For this review, take the finished solid that the model builds, in its own axes (mm). A direction names the side the tool comes from. Coordinates: 2 decimals unless noted, no trailing zeros. Loops run counter-clockwise (first coordinate to the right, second up) from the corner with the lowest first, then second, coordinate; pieces in that order, holes last. Notation, with made-up numbers: (61, -9.75) - (68, -9.75) arc R30 cw to (68, 19.25) - close; hole circle Ø4 at (-5.5, 17.25). An arc over 180 degrees is marked (long way). One line per item, written item: value. Start each with the question number.
1. To check wall thickness, follow line 1 (Y direction, x = 0.25, z = 0); line 2 (X direction, y = 3, z = -10); line 3 (X direction, y = 5, z = -1.5). State the ranges of each line that lie inside material, in increasing order. Write a range as from..to.
2. The part is to be moulded in two halves that separate along Z. For faces 4 (the face through (10.8, 17.25, 2.27)), 5 (the face through (0.49, 6.31, 20.03)), 6 (the face through (0, -20, 7)), say which applies: released by +Z, released by -Z, zero draft, split by the parting line, or undercut.
3. For faces 1 (the face through (2, 0, 0)), 2 (the face through (17, 0, 0)), 3 (the face through (13.479, 8.923, 1.172)), list the 3-axis set-ups (+Z, -Z, +X, -X, +Y, -Y) from which the entire face can be reached by the end or side of a thin tool; tool diameter is ignored.
4. Take a section at B-B, the plane x = 10.5. State the section outline as (y, z) points, and give its area (3 significant figures).
5. Take a section at A-A, the plane z = 0. State the section outline as (x, y) points.
6. Insertion check: pin 1 (6 mm diameter, centred on x = 2.5, y = -9.5, fed in from -Z); pin 2 (4 mm diameter, centred on x = 9, z = 5, fed in from -Y); pin 3 (2 mm diameter, centred on y = -17, z = 2.5, fed in from -X). Each pin has a flat end and moves straight along its axis. Give the tip position at first contact, or say it passes through.
```python
from build123d import *

# Parameters (mm, degrees)
SKETCH1_R           = 22.5
BOSS_EXTRUDE1_DEPTH = 3
SKETCH3_R           = 17
SKETCH2_R           = 20
SKETCH4_R           = 9
BOSS_EXTRUDE2_DEPTH = 5
FILLET1_R           = 2
FILLET2_R           = 1
SKETCH5_R           = 21
CUT_EXTRUDE1_DEPTH  = 2
BOSS_EXTRUDE3_START = 1
SKETCH6_R           = 21
SKETCH6_R_2         = 16
BOSS_EXTRUDE3_DEPTH = 1
FILLET3_R           = 6


with BuildPart() as part:
    # Sketch1 → Boss-Extrude1 (new body)
    with BuildSketch(Plane(origin=(0, 0, 0), x_dir=(0, 0, -1), z_dir=(1, 0, 0))):
        Circle(SKETCH1_R)
    extrude(amount=BOSS_EXTRUDE1_DEPTH)

    # Sketch3 → Loft1 section 0
    with BuildSketch(Plane(origin=(12, 0, 0), x_dir=(0, 0, -1), z_dir=(1, 0, 0))):
        Circle(SKETCH3_R)
    # Sketch2 → Loft1 section 1
    with BuildSketch(Plane(origin=(3, 0, 0), x_dir=(0, 0, -1), z_dir=(1, 0, 0))):
        Circle(SKETCH2_R)
    loft()

    # Sketch4 → Boss-Extrude2 (add)
    with BuildSketch(Plane(origin=(12, 0, 0), x_dir=(0, 0, -1), z_dir=(1, 0, 0))):
        Circle(SKETCH4_R)
    extrude(amount=BOSS_EXTRUDE2_DEPTH)

    # Fillet1
    fillet1_edges = [part.edges().sort_by_distance(p)[0] for p in [
        (17, 0, 9),
    ]]
    fillet(fillet1_edges, radius=FILLET1_R)

    # Fillet2
    fillet2_edges = [part.edges().sort_by_distance(p)[0] for p in [
        (3, 0, 22.5),
        (12, 0, 17),
    ]]
    fillet(fillet2_edges, radius=FILLET2_R)

    # Sketch5 → Cut-Extrude1 (cut)
    with BuildSketch(Plane.ZY):
        Circle(SKETCH5_R)
    extrude(amount=-CUT_EXTRUDE1_DEPTH, mode=Mode.SUBTRACT)

    # Sketch6 → Boss-Extrude3 (add)
    with BuildSketch(Plane.ZY.offset(-2).offset(BOSS_EXTRUDE3_START)):
        Circle(SKETCH6_R)
        Circle(SKETCH6_R_2, mode=Mode.SUBTRACT)
    extrude(amount=-BOSS_EXTRUDE3_DEPTH)

    # Fillet3
    # the kernel refuses this fillet: 6 mm, written as the material it takes off along each edge
    with BuildSketch(Plane(origin=(1, 0, 0), x_dir=(0, 0, 1), z_dir=(0, -1, 0))) as fillet3_piece_1:
        with BuildLine():
            CenterArc((19.31662479, -6), FILLET3_R, 90, 33.557309762)
            Line((16, -1), (16, 0))
            Line((16, 0), (19.31662479, 0))
        make_face()
    revolve(axis=Axis((1, 0, 0), (-1, 0, 0)), mode=Mode.SUBTRACT)


solid = part.part
```
Solutions:
1. line 1: -22.5..-21, 21..22.5
1. line 2: 2..12
1. line 3: 2..17
2. face 4: split by the parting line
2. face 5: undercut
2. face 6: zero draft
3. face 1: -X
3. face 2: +Z, -Z, +X, +Y, -Y
3. face 3: +X
4. outline: circle Ø35 at (0, 0)
4. area: 962 mm2
5. outline: (0, -22.5) - (2, -22.5) arc R1 ccw to (3, -21.5) - (3, -20) - (11.32, -17.23) arc R1 ccw to (12, -16.28) - (12, -9) - (15, -9) arc R2 ccw to (17, -7) - (17, 7) arc R2 ccw to (15, 9) - (12, 9) - (12, 16.28) arc R1 ccw to (11.32, 17.23) - (3, 20) - (3, 21.5) arc R1 ccw to (2, 22.5) - (0, 22.5) - (0, 21) - (1, 21) - (1, 19.32) arc R6 ccw to (2, 16) - (2, -16) arc R6 ccw to (1, -19.32) - (1, -21) - (0, -21) - close
6. pin 1: z = -21.53
6. pin 2: y = -18.14
6. pin 3: x = 1.11
